from build123d import *

# Parameters (mm, degrees)
SKETCH_R         = 2.1
PAD_DEPTH        = 1000
CHAMFER_1_ANGLE  = 45
CHAMFER_1_SIZE   = 1.7
CHAMFER_2_ANGLE  = 45
CHAMFER_2_SIZE   = 1.7
CHAMFER_3_ANGLE  = 45
CHAMFER_3_SIZE   = 1.7
CHAMFER_4_ANGLE  = 45
CHAMFER_4_SIZE   = 1.7
CHAMFER_5_ANGLE  = 45
CHAMFER_5_SIZE   = 1.7
CHAMFER_6_ANGLE  = 45
CHAMFER_6_SIZE   = 1.7
CHAMFER_7_ANGLE  = 45
CHAMFER_7_SIZE   = 1.7
CHAMFER_8_ANGLE  = 45
CHAMFER_8_SIZE   = 1.7
CHAMFER_9_ANGLE  = 45
CHAMFER_9_SIZE   = 1.7
CHAMFER_10_ANGLE = 45
CHAMFER_10_SIZE  = 1.7
CHAMFER_11_ANGLE = 45
CHAMFER_11_SIZE  = 1.7
CHAMFER_12_ANGLE = 45
CHAMFER_12_SIZE  = 1.7
FILLET_R         = 0.2


with BuildPart() as part:
    # Sketch → Pad (new body)
    with BuildSketch(Plane.XY):
        Polygon((0, 3.723883), (0.176777, 3.90066), (2.84, 3.90066), (5.49934, 6.56), (5.49934, 8.2), (3.1, 8.2), (3.1, 10), (16.9, 10), (16.9, 8.2), (14.50066, 8.2), (14.50066, 6.56), (17.16, 3.90066), (19.823223, 3.90066), (20, 3.723883), (20.176777, 3.90066), (22.84, 3.90066), (25.49934, 6.56), (25.49934, 8.2), (23.1, 8.2), (23.1, 10), (30, 10), (30, 3.1), (28.2, 3.1), (28.2, 5.49934), (26.56, 5.49934), (23.90066, 2.84), (23.90066, 0.176777), (23.723883, 0), (23.90066, -0.176777), (23.90066, -2.84), (26.56, -5.49934), (28.2, -5.49934), (28.2, -3.1), (30, -3.1), (30, -10), (23.1, -10), (23.1, -8.2), (25.49934, -8.2), (25.49934, -6.56), (22.84, -3.90066), (20.176777, -3.90066), (20, -3.723883), (19.823223, -3.90066), (17.16, -3.90066), (14.50066, -6.56), (14.50066, -8.2), (16.9, -8.2), (16.9, -10), (3.1, -10), (3.1, -8.2), (5.49934, -8.2), (5.49934, -6.56), (2.84, -3.90066), (0.176777, -3.90066), (0, -3.723883), (-0.176777, -3.90066), (-2.84, -3.90066), (-5.49934, -6.56), (-5.49934, -8.2), (-3.1, -8.2), (-3.1, -10), (-10, -10), (-10, -3.1), (-8.2, -3.1), (-8.2, -5.49934), (-6.56, -5.49934), (-3.90066, -2.84), (-3.90066, -0.176777), (-3.723883, 0), (-3.90066, 0.176777), (-3.90066, 2.84), (-6.56, 5.49934), (-8.2, 5.49934), (-8.2, 3.1), (-10, 3.1), (-10, 10), (-3.1, 10), (-3.1, 8.2), (-5.49934, 8.2), (-5.49934, 6.56), (-2.84, 3.90066), (-0.176777, 3.90066), align=None)
        Circle(SKETCH_R, mode=Mode.SUBTRACT)
        with Locations((20, 0)):
            Circle(SKETCH_R, mode=Mode.SUBTRACT)
        Polygon((7.29934, 6.23868), (3.90066, 2.84), (3.90066, 0.176777), (3.723883, 0), (3.90066, -0.176777), (3.90066, -2.84), (7.29934, -6.23868), (7.29934, -8.2), (12.70066, -8.2), (12.70066, -6.23868), (16.09934, -2.84), (16.09934, -0.176777), (16.276117, 0), (16.09934, 0.176777), (16.09934, 2.84), (12.70066, 6.23868), (12.70066, 8.2), (7.29934, 8.2), align=None, mode=Mode.SUBTRACT)
    extrude(amount=PAD_DEPTH)

    # Chamfer 1
    chamfer_1_edges = [part.edges().sort_by_distance(p)[0] for p in [
        (3.1, -10, 500),
    ]]
    chamfer_1_side = part.faces().sort_by_distance((10, -10, 500))[0]
    chamfer(chamfer_1_edges, length=CHAMFER_1_SIZE, angle=CHAMFER_1_ANGLE, reference=chamfer_1_side)

    # Chamfer 2
    chamfer_2_edges = [part.edges().sort_by_distance(p)[0] for p in [
        (16.9, -10, 500),
    ]]
    chamfer_2_side = part.faces().sort_by_distance((16.9, -9.1, 500))[0]
    chamfer(chamfer_2_edges, length=CHAMFER_2_SIZE, angle=CHAMFER_2_ANGLE, reference=chamfer_2_side)

    # Chamfer 3
    chamfer_3_edges = [part.edges().sort_by_distance(p)[0] for p in [
        (23.1, -10, 500),
    ]]
    chamfer_3_side = part.faces().sort_by_distance((26.55, -10, 500))[0]
    chamfer(chamfer_3_edges, length=CHAMFER_3_SIZE, angle=CHAMFER_3_ANGLE, reference=chamfer_3_side)

    # Chamfer 4
    chamfer_4_edges = [part.edges().sort_by_distance(p)[0] for p in [
        (-3.1, -10, 500),
    ]]
    chamfer_4_side = part.faces().sort_by_distance((-3.1, -9.1, 500))[0]
    chamfer(chamfer_4_edges, length=CHAMFER_4_SIZE, angle=CHAMFER_4_ANGLE, reference=chamfer_4_side)

    # Chamfer 5
    chamfer_5_edges = [part.edges().sort_by_distance(p)[0] for p in [
        (30, -3.1, 500),
    ]]
    chamfer_5_side = part.faces().sort_by_distance((29.1, -3.1, 500))[0]
    chamfer(chamfer_5_edges, length=CHAMFER_5_SIZE, angle=CHAMFER_5_ANGLE, reference=chamfer_5_side)

    # Chamfer 6
    chamfer_6_edges = [part.edges().sort_by_distance(p)[0] for p in [
        (30, 3.1, 500),
    ]]
    chamfer_6_side = part.faces().sort_by_distance((30, 6.55, 500))[0]
    chamfer(chamfer_6_edges, length=CHAMFER_6_SIZE, angle=CHAMFER_6_ANGLE, reference=chamfer_6_side)

    # Chamfer 7
    chamfer_7_edges = [part.edges().sort_by_distance(p)[0] for p in [
        (23.1, 10, 500),
    ]]
    chamfer_7_side = part.faces().sort_by_distance((23.1, 9.1, 500))[0]
    chamfer(chamfer_7_edges, length=CHAMFER_7_SIZE, angle=CHAMFER_7_ANGLE, reference=chamfer_7_side)

    # Chamfer 8
    chamfer_8_edges = [part.edges().sort_by_distance(p)[0] for p in [
        (16.9, 10, 500),
    ]]
    chamfer_8_side = part.faces().sort_by_distance((10, 10, 500))[0]
    chamfer(chamfer_8_edges, length=CHAMFER_8_SIZE, angle=CHAMFER_8_ANGLE, reference=chamfer_8_side)

    # Chamfer 9
    chamfer_9_edges = [part.edges().sort_by_distance(p)[0] for p in [
        (3.1, 10, 500),
    ]]
    chamfer_9_side = part.faces().sort_by_distance((3.1, 9.1, 500))[0]
    chamfer(chamfer_9_edges, length=CHAMFER_9_SIZE, angle=CHAMFER_9_ANGLE, reference=chamfer_9_side)

    # Chamfer 10
    chamfer_10_edges = [part.edges().sort_by_distance(p)[0] for p in [
        (-3.1, 10, 500),
    ]]
    chamfer_10_side = part.faces().sort_by_distance((-6.55, 10, 500))[0]
    chamfer(chamfer_10_edges, length=CHAMFER_10_SIZE, angle=CHAMFER_10_ANGLE, reference=chamfer_10_side)

    # Chamfer 11
    chamfer_11_edges = [part.edges().sort_by_distance(p)[0] for p in [
        (-10, -3.1, 500),
    ]]
    chamfer_11_side = part.faces().sort_by_distance((-10, -6.55, 500))[0]
    chamfer(chamfer_11_edges, length=CHAMFER_11_SIZE, angle=CHAMFER_11_ANGLE, reference=chamfer_11_side)

    # Chamfer 12
    chamfer_12_edges = [part.edges().sort_by_distance(p)[0] for p in [
        (-10, 3.1, 500),
    ]]
    chamfer_12_side = part.faces().sort_by_distance((-9.1, 3.1, 500))[0]
    chamfer(chamfer_12_edges, length=CHAMFER_12_SIZE, angle=CHAMFER_12_ANGLE, reference=chamfer_12_side)

    # Fillet
    fillet_edges = [part.edges().sort_by_distance(p)[0] for p in [
        (-10, -10, 500),
        (-10, 10, 500),
        (30, 10, 500),
        (30, -10, 500),
    ]]
    fillet(fillet_edges, radius=FILLET_R)


solid = part.part
Verification items for the finished model (mm, model axes). Give positions to 0.01 mm unless a question says otherwise; leave off trailing zeros.
(1) Cross-section at A-A (z = 790). State how many separate pieces and enclosed holes the cut face has, plus the area to 3 significant figures.
(2) Material ranges on line 1 (X direction, y = -0.5, z = 114); line 2 (X direction, y = -4.75, z = 496.5); line 3 (Y direction, x = 0.5, z = 913.5), recorded low to high.
(3) Gauge pin test, flat ends, axial feed: pin 1 (1.2 mm diameter, centred on y = -4, z = 501.5, fed in from +X); pin 2 (1.3 mm diameter, centred on x = 1.5, z = 275.5, fed in from -Y); pin 3 (1.3 mm diameter, centred on y = -1, z = 494.5, fed in from +X). Record the tip position at first contact, or that the pin passes through.
Worked out:
1. separate pieces: 1
1. enclosed holes: 3
1. area: 296 mm2
2. line 1: x = -3.9 to -2.04, 2.04 to 3.9, 16.1 to 17.96, 22.04 to 23.9
2. line 2: x = -9.95 to -8.2, -5.81 to -3.69, 3.69 to 5.81, 14.19 to 16.31, 23.69 to 25.81, 28.2 to 29.95
2. line 3: y = -3.9 to -2.04, 2.04 to 3.9
3. pin 1: stops at x = 29.8
3. pin 2: stops at y = -3.9
3. pin 3: stops at x = 23.9
